Build history of the part. All positions in model axes, mm. A direction names the side the tool comes from. Round coordinates to 2 decimals unless told otherwise and drop trailing zeros. Order: outer loops, then holes, each group sorted by start corner. A loop starts at its lowest first (then second) coordinate and runs counter-clockwise, first axis right, second up. Notation, with made-up numbers: M -25.75,-10.5 L 22.25,-10.5 A13 ccw 22.25,-5.5 Z; hole C -24.5,45.5 d1. An arc over 180 degrees is marked long. Use CSV: the item, a comma, the result in double quotes.
from build123d import *

# Parameters (mm, degrees)
SKETCH1_W               = 8
SKETCH1_H               = 8
BOSS_EXTRUDE1_DEPTH     = 3
CUT_EXTRUDE1_DEPTH      = 12.704699911
CUT_EXTRUDE1_DEPTH_BACK = 12.704699911
CUT_EXTRUDE2_DEPTH      = 11
SKETCH4_R               = 1.75
CUT_EXTRUDE3_DEPTH      = 0.4
SKETCH5_W               = 8
SKETCH5_H               = 1
BOSS_EXTRUDE2_DEPTH     = 2
FILLET1_R               = 4
CUT_EXTRUDE4_DEPTH      = 0.4


with BuildPart() as part:
    # Sketch1 → Boss-Extrude1 (new body)
    with BuildSketch(Plane(origin=(0, 0, 0), x_dir=(1, 0, 0), z_dir=(0, 1, 0))):
        with Locations((4, 4)):
            Rectangle(SKETCH1_W, SKETCH1_H)
    extrude(amount=BOSS_EXTRUDE1_DEPTH)

    # Sketch2 → Cut-Extrude1 (cut, two sides: drawn at the far end of the back side and taken through both)
    with BuildSketch(Plane.XY.offset(-CUT_EXTRUDE1_DEPTH_BACK)):
        Polygon((0, 0), (0.6, 3), (0, 3), align=None)
        Polygon((8, 0), (7.4, 3), (8, 3), align=None)
    extrude(amount=CUT_EXTRUDE1_DEPTH + CUT_EXTRUDE1_DEPTH_BACK, mode=Mode.SUBTRACT)

    # Sketch3 → Cut-Extrude2 (cut)
    with BuildSketch(Plane(origin=(0, 0, 0), x_dir=(0, 0, -1), z_dir=(1, 0, 0))):
        Polygon((0, 0), (0.6, 3), (0, 3), align=None)
        Polygon((8, 3), (7.4, 3), (8, 0), align=None)
    extrude(amount=CUT_EXTRUDE2_DEPTH, mode=Mode.SUBTRACT)

    # Sketch4 → Cut-Extrude3 (cut)
    with BuildSketch(Plane.XZ):
        with Locations(Location((4, -3.75, 0), (0, 0, 270))):
            Circle(SKETCH4_R)
    extrude(amount=-CUT_EXTRUDE3_DEPTH, mode=Mode.SUBTRACT)

    # Sketch5 → Boss-Extrude2 (add)
    with BuildSketch(Plane.XZ):
        with Locations((4, -7.5)):
            Rectangle(SKETCH5_W, SKETCH5_H)
    extrude(amount=BOSS_EXTRUDE2_DEPTH)

    # Fillet1
    # the kernel refuses this fillet: 4 mm, written as the material it takes off along each edge
    with BuildSketch(Plane(origin=(8, -2, -16.660254038), x_dir=(0, 1, 0), z_dir=(0, 0, 1)), Plane(origin=(0, -2, 1.660254038), x_dir=(0, 1, 0), z_dir=(0, 0, -1))) as fillet1_piece_1:
        with BuildLine():
            CenterArc((4, 3.464101615), FILLET1_R, 180, 60)
            Line((0, 3.464101615), (-0.08, 3.464101615))
            Line((-0.08, 3.464101615), (-0.08, 0))
            Line((-0.08, 0), (0, -0.08))
            ThreePointArc((0, -0.08), (1, -0.08), (1.96, -0.069282032))
            Line((1.96, -0.069282032), (2, 0))
        make_face()
    extrude(amount=18.320508076, mode=Mode.SUBTRACT)

    # Sketch6 → Cut-Extrude4 (cut)
    with BuildSketch(Plane(origin=(0, 3, 0), x_dir=(1, 0, 0), z_dir=(0, 1, 0))):
        with BuildLine():
            Line((4.984953699, 3.505457585), (5.754184468, 3.249047329))
            add(Edge.make_bspline(
                [(5.754184468, 3.249047329), (5.738551331, 3.198610805), (5.707936732, 3.099840225), (5.651723194, 2.958278532), (5.587443886, 2.827086856), (5.517410433, 2.704729688), (5.437267593, 2.594367909), (5.351502188, 2.492347505), (5.25756407, 2.400817223), (5.155916755, 2.319581611), (5.047538657, 2.247743191), (4.931170847, 2.187011676), (4.808549951, 2.134705195), (4.678432524, 2.092325917), (4.541682112, 2.058386549), (4.397657073, 2.035969411), (4.247031142, 2.020769852), (4.144181592, 2.01912185), (4.091524212, 2.018278098)],
                knots=[0, 0, 0, 0, 1.126640671, 2.206316847, 3.246446654, 4.24268115, 5.210795778, 6.153057602, 7.084219323, 8.004711971, 8.926421631, 9.854560063, 10.802134612, 11.768317461, 12.772025444, 13.805668576, 14.876536225, 16, 16, 16, 16], degree=3))
            add(Edge.make_bspline(
                [(4.091524212, 2.018278098), (4.026529436, 2.019622049), (3.898682769, 2.022265641), (3.711719127, 2.048877042), (3.533551231, 2.090397174), (3.363924198, 2.147881075), (3.203970267, 2.224018355), (3.052230113, 2.31567777), (2.909808045, 2.424720155), (2.777203704, 2.549307725), (2.656729454, 2.688489389), (2.552550394, 2.841513049), (2.46353299, 3.006222974), (2.391584534, 3.18340452), (2.335325697, 3.372875751), (2.295916265, 3.574374695), (2.271256348, 3.787964822), (2.268446864, 3.934340923), (2.267004981, 4.009463995)],
                knots=[0, 0, 0, 0, 1.025049111, 2.016302254, 2.973197159, 3.90886983, 4.83646737, 5.763135642, 6.70136783, 7.661478232, 8.629732022, 9.600038443, 10.576877021, 11.5787097, 12.612181225, 13.690866959, 14.814907849, 16, 16, 16, 16], degree=3))
            add(Edge.make_bspline(
                [(2.267004981, 4.009463995), (2.268440364, 4.088592426), (2.271240535, 4.242957555), (2.295946649, 4.467391238), (2.33430142, 4.6789069), (2.390655342, 4.87619306), (2.461546504, 5.060638151), (2.550671985, 5.230411199), (2.653811862, 5.387775744), (2.773739341, 5.529847487), (2.90694801, 5.655987983), (3.049697575, 5.767530284), (3.203319761, 5.861106277), (3.366973913, 5.937627827), (3.540879519, 5.996843969), (3.724694381, 6.039484239), (3.918568892, 6.064303618), (4.051121857, 6.067784001), (4.118767802, 6.069560149)],
                knots=[0, 0, 0, 0, 1.212648312, 2.365655595, 3.457000981, 4.504219827, 5.506356588, 6.480637568, 7.437950897, 8.385265166, 9.323599949, 10.245787653, 11.157260172, 12.074946661, 13.00980897, 13.968233668, 14.963125779, 16, 16, 16, 16], degree=3))
            add(Edge.make_bspline(
                [(4.118767802, 6.069560149), (4.177845619, 6.068071541), (4.293675542, 6.065152928), (4.463296702, 6.045323759), (4.624050093, 6.010524892), (4.776804639, 5.963554159), (4.920690778, 5.901565287), (5.05596628, 5.825815524), (5.18309612, 5.736705664), (5.259694467, 5.667100309), (5.298254981, 5.632060149)],
                knots=[0, 0, 0, 0, 1.098510076, 2.153775193, 3.169777012, 4.153122333, 5.120892526, 6.076995459, 7.031936742, 8, 8, 8, 8], degree=3))
            add(Edge.make_bspline(
                [(5.298254981, 5.632060149), (5.320604149, 5.60976374), (5.365827451, 5.564647194), (5.426213252, 5.488477681), (5.483466493, 5.406481188), (5.536678451, 5.317258958), (5.58416733, 5.220136739), (5.628218337, 5.11660602), (5.668774447, 5.006267724), (5.691328308, 4.929479087), (5.702902417, 4.89007297)],
                knots=[0, 0, 0, 0, 0.885292881, 1.791380647, 2.722937556, 3.69093542, 4.703306561, 5.754477758, 6.847650944, 8, 8, 8, 8], degree=3))
            Line((5.702902417, 4.89007297), (4.933671648, 4.736226816))
            add(Edge.make_bspline(
                [(4.933671648, 4.736226816), (4.927133502, 4.76145763), (4.914255072, 4.811155713), (4.888197319, 4.88256913), (4.858307022, 4.950334085), (4.821260737, 5.012790777), (4.781908002, 5.072717729), (4.735316585, 5.127453998), (4.684461977, 5.178434101), (4.62897783, 5.22512899), (4.569525593, 5.266595122), (4.507249934, 5.303870591), (4.441018967, 5.334299022), (4.371713727, 5.358915551), (4.29961025, 5.379554656), (4.224066596, 5.392304393), (4.145731594, 5.40209207), (4.092359182, 5.40262243), (4.065081904, 5.402893482)],
                knots=[0, 0, 0, 0, 1.051226935, 2.070641259, 3.064374968, 4.034983734, 4.997599858, 5.953980297, 6.92954377, 7.901109626, 8.875958313, 9.851998019, 10.826131395, 11.811470594, 12.818270757, 13.847890818, 14.900111925, 16, 16, 16, 16], degree=3))
            add(Edge.make_bspline(
                [(4.065081904, 5.402893482), (4.027621622, 5.402136956), (3.95451036, 5.400660441), (3.84764705, 5.384198307), (3.745794169, 5.361223694), (3.649362485, 5.32614158), (3.558949174, 5.281271846), (3.473526684, 5.226727667), (3.393563858, 5.162742669), (3.319033671, 5.088558841), (3.252152959, 5.002834902), (3.193355266, 4.905393862), (3.144577309, 4.795129453), (3.104977365, 4.673123713), (3.073807698, 4.539086512), (3.051550102, 4.39284594), (3.039240982, 4.234301954), (3.037259111, 4.124602201), (3.03623575, 4.067957585)],
                knots=[0, 0, 0, 0, 0.938194206, 1.831074359, 2.704771284, 3.551924377, 4.396294915, 5.230222094, 6.087631332, 6.958733431, 7.860107878, 8.806247581, 9.804197948, 10.875520245, 12.017191412, 13.250061517, 14.580040491, 16, 16, 16, 16], degree=3))
            add(Edge.make_bspline(
                [(3.03623575, 4.067957585), (3.037249034, 4.007841988), (3.039201475, 3.892008492), (3.051507983, 3.724929387), (3.073907907, 3.571260811), (3.104663329, 3.430730056), (3.144462832, 3.303423199), (3.1931583, 3.189560541), (3.251047919, 3.089008738), (3.318041624, 3.001834743), (3.3924457, 2.926952551), (3.472244969, 2.862570915), (3.55696863, 2.80752487), (3.647126515, 2.762236533), (3.743061533, 2.72797641), (3.843985242, 2.703130369), (3.950267946, 2.687335345), (4.023091528, 2.685752793), (4.060274212, 2.684944765)],
                knots=[0, 0, 0, 0, 1.475208372, 2.842499301, 4.107722225, 5.282836115, 6.369007568, 7.375918121, 8.315702116, 9.208439171, 10.065831443, 10.90006451, 11.71996243, 12.54067204, 13.369972975, 14.214060185, 15.088124569, 16, 16, 16, 16], degree=3))
            add(Edge.make_bspline(
                [(4.060274212, 2.684944765), (4.087802914, 2.685631562), (4.141934021, 2.686982048), (4.22194397, 2.695553476), (4.298737204, 2.711910812), (4.3726896, 2.733540427), (4.444088489, 2.760679214), (4.511844803, 2.795492821), (4.577291618, 2.835505891), (4.639070965, 2.882398144), (4.6980101, 2.93504365), (4.751766089, 2.995888735), (4.801629231, 3.063471428), (4.846966938, 3.138243387), (4.889294086, 3.219564589), (4.92530624, 3.308702064), (4.958854788, 3.404215308), (4.976102112, 3.471120718), (4.984953699, 3.505457585)],
                knots=[0, 0, 0, 0, 0.980177776, 1.927374078, 2.859849964, 3.771585772, 4.668674471, 5.574490016, 6.479656464, 7.396337719, 8.332153134, 9.288470092, 10.28125149, 11.318486971, 12.398724812, 13.541284404, 14.738150009, 16, 16, 16, 16], degree=3))
        make_face()
    extrude(amount=-CUT_EXTRUDE4_DEPTH, mode=Mode.SUBTRACT)


solid = part.part
(1) Two-plate mould, pull along X, no slides. Class faces 1 (the face through (0.3, 1.5, -4.1)), 2 (the face through (4, -1, -8)), 3 (the face through (4, 0.4, -4)): released by +X, released by -X, zero draft, split by the parting line, or undercut.
Answer block:
face 1,"released by -X"
face 2,"zero draft"
face 3,"undercut"
(2) Cut at D-D, the plane x = 1.25. Give the cut face in (y, z).
Answer block:
outline,"M -1.33,-8 L 0,-8 L 3,-7.4 L 3,-0.6 L 0,0 L 0,-7 L -1.33,-7 Z"
(3) Cut at A-A, the plane y = 0.95. Give the cut face in (x, z).
Answer block:
outline,"M 0.19,-7.81 L 7.81,-7.81 L 7.81,-0.19 L 0.19,-0.19 Z"
(4) Drop flat-ended pins along their axis: pin 1 (2 mm diameter, centred on x = 2.5, z = -4, fed in from -Y); pin 2 (1 mm diameter, centred on x = 5.5, y = -1, fed in from +Z); pin 3 (1.6 mm diameter, centred on x = 6, y = -0.5, fed in from +Z); pin 4 (1 mm diameter, centred on y = 1.5, z = -7, fed in from +X). Give the stop position or say it passes through.
Answer block:
pin 1,"stops at y = 0"
pin 2,"stops at z = -7"
pin 3,"stops at z = 0"
pin 4,"stops at x = 7.8"
(5) Cut at B-B, the plane x = 6.5. Give the cut face in (y, z), and give its area (3 significant figures).
Answer block:
outline,"M -1.48,-8 L 0,-8 L 3,-7.4 L 3,-0.6 L 0,0 L 0,-7 L -1.48,-7 Z"
area,"23.7 mm²"
(6) Wall check: line 1 (Y direction, x = 3.25, z = -6.5); line 2 (Y direction, x = 3, z = -3.5); line 3 (Z direction, x = 4.25, y = 2.8). Give the ranges that are in metal, low to high. Write a range as from..to.
Answer block:
line 1,"y = 0..3"
line 2,"y = 0.4..2.6"
line 3,"z = -7.44..-6.07, -5.39..-2.7, -2.02..-0.56"
(7) Tool access for faces 4 (the face through (4, -2, -7.5)), 5 (the face through (3, 0, -2)), 6 (the face through (2.87, 2.6, -4.07)), 7 (the face through (2.94, 0.2, -2.36)), 8 (the face through (4, 3, -4)): list every direction of +Z, -Z, +X, -X, +Y, -Y with a clear straight run to the whole face (end or side of a thin tool).
Answer block:
face 4,"+Z, -Z, +X, -X, -Y"
face 5,"+Z, +X, -X, -Y"
face 6,"+Y"
face 7,"-Y"
face 8,"+Z, -Z, +X, -X, +Y"
(8) Cut at C-C, the plane z = -6.25. Give the cut face in (x, y).
Answer block:
outline,"M 0,0 L 8,0 L 7.4,3 L 0.6,3 Z"
